Here's how the part is built. I have some questions about the finished solid (model axes, mm). A direction names the side the tool comes from. Give positions to 0.01 mm unless a question says otherwise; leave off trailing zeros. Loops run counter-clockwise (first coordinate to the right, second up) from the corner with the lowest first, then second, coordinate; pieces in that order, holes last.
Q1. Suppose I cut it at A-A (z = -38.5). List the corners of the cut face in (x, y) for me.
Q2. I need wall thicknesses on probe 1 along Y at (x, z) = (0, -36.25); probe 2 along Y at (x, z) = (0, 24); probe 3 along X at (y, z) = (-18.5, -32). Which ranges of each line are inside material? Lowest first, please.
Q3. Suppose I cut it at B-B (z = -15.5). List the corners of the cut face in (x, y) for me.
Q4. I'm going to push flat-ended pins straight in: P1, Ø1, axis at y = -40.5, z = -13.5, coming from the -X side; P2, Ø1, axis at x = 27, z = -35.5, coming from the -Y side; P3, Ø8, axis at x = -73.5, z = -31.5, coming from the +Y side. Where does each tip first touch, or does it pass through?
Q5. For faces 1 (the face through (19.635, 88.423, 1.325)), 2 (the face through (9.764, 74.362, -39.64)), 3 (the face through (-28, -21, 40)), which set-ups out of +Z, -Z, +X, -X, +Y, -Y let a thin tool reach every point of the face, with its end or its side?
Q6. Thinking about a two-plate mould opening in Z: for faces 4 (the face through (19.635, 88.423, 26.325)), 5 (the face through (-24, 8, -49.5)), 6 (the face through (-9.764, 74.362, 39.64)), 7 (the face through (14, 74, 49.5)), which applies, pulls with the +Z half, pulls with the -Z half, needs draft (parallel to the pull), parting line crosses it, or undercut?
```python
from build123d import *

# Parameters (mm, degrees)
SKETCH1_R               = 99.5
BOSS_EXTRUDE1_DEPTH     = 49.5
SKETCH3_R               = 75
SKETCH3_R_2             = 35
CUT_EXTRUDE1_DEPTH      = 20
SKETCH4_R               = 25
CUT_EXTRUDE2_DEPTH      = 1.0000001
CUT_EXTRUDE2_DEPTH_BACK = 100.0000001
SKETCH5_R               = 75
SKETCH5_R_2             = 35
CUT_EXTRUDE3_DEPTH      = 20


with BuildPart() as part:
    # Sketch1 → Boss-Extrude1 (new body, symmetric)
    with BuildSketch(Plane.XY):
        Circle(SKETCH1_R)
    extrude(amount=BOSS_EXTRUDE1_DEPTH, both=True)

    # Sketch2 → Cut-Revolve1 (revolve, cut)
    with BuildSketch(Plane(origin=(0, 0, 0), x_dir=(1, 0, 0), z_dir=(0, 1, 0))):
        Polygon((-89.981945933, -25.982850646), (-99.911722122, -31.694962561), (-99.915568006, -18.158689934), (-90.018054068, -23.893839429), align=None)
        Polygon((-89.981945933, -0.982850646), (-99.911722122, -6.694962562), (-99.92977619, 6.849543049), (-90.018054068, 1.106160571), align=None)
        Polygon((-90.016592149, 23.99721909), (-99.911722122, 18.305037438), (-99.92977619, 31.849543049), (-90.018054068, 26.106160571), align=None)
    revolve(axis=Axis((0, 0, 0), (0, 0, 1)), mode=Mode.SUBTRACT)

    # Sketch3 → Cut-Extrude1 (cut)
    with BuildSketch(Plane(origin=(0, 0, -49.5), x_dir=(-1, 0, 0), z_dir=(0, 0, -1))):
        Circle(SKETCH3_R)
        Circle(SKETCH3_R_2, mode=Mode.SUBTRACT)
    extrude(amount=-CUT_EXTRUDE1_DEPTH, mode=Mode.SUBTRACT)

    # Sketch4 → Cut-Extrude2 (cut, two sides)
    with BuildSketch(Plane.XY.offset(49.5)) as cut_extrude2_sk:
        Circle(SKETCH4_R)
    extrude(amount=CUT_EXTRUDE2_DEPTH, mode=Mode.SUBTRACT)
    extrude(cut_extrude2_sk.sketch, amount=-CUT_EXTRUDE2_DEPTH_BACK, mode=Mode.SUBTRACT)

    # Sketch5 → Cut-Extrude3 (cut)
    with BuildSketch(Plane.XY.offset(49.5)):
        Circle(SKETCH5_R)
        Circle(SKETCH5_R_2, mode=Mode.SUBTRACT)
    extrude(amount=-CUT_EXTRUDE3_DEPTH, mode=Mode.SUBTRACT)


solid = part.part
```
Solutions:
1. outline: circle Ø199 at (0, 0); circle Ø70 at (0, 0); hole circle Ø150 at (0, 0); hole circle Ø50 at (0, 0)
2. probe 1: y = -99.5 to -75, -35 to -25, 25 to 35, 75 to 99.5
2. probe 2: y = -90.02 to -25, 25 to 90.02
2. probe 3: x = -97.77 to -72.68, -29.71 to -16.82, 16.82 to 29.71, 72.68 to 97.77
3. outline: circle Ø199 at (0, 0); hole circle Ø50 at (0, 0)
4. P1: stops at x = -91.11
4. P2: stops at y = -95.91
4. P3: stops at y = 71.2
5. face 1: none
5. face 2: -Z
5. face 3: +Z
6. face 4: undercut
6. face 5: pulls with the -Z half
6. face 6: needs draft
6. face 7: pulls with the +Z half
